```python
from build123d import *

# Parameters (mm, degrees)
F1_DEPTH = 63.5
F0_W     = 25.4
F0_H     = 19.05
F2_DEPTH = 25.4
F3_DEPTH = 7.9375
F5_R     = 6.35


with BuildPart() as f1:
    # F0 (on Front) → F1 (new body, symmetric)
    with BuildSketch(Plane.XZ):
        Polygon((41.275, -9.525), (41.275, 9.525), (22.225, 9.525), (-41.275, 9.525), (-41.275, -9.525), align=None)
    extrude(amount=F1_DEPTH, both=True)

    # F0 (on Front) → F2 (join, symmetric)
    with BuildSketch(Plane.XZ):
        with BuildLine():
            Line((57.15, 42.8752), (60.325, 42.8752))
            Line((60.325, 42.8752), (60.325, 61.9252))
            Line((60.325, 61.9252), (57.15, 61.9252))
            add(Edge.make_bspline(
                [(55.1509005081, 61.8679390466), (55.8211077358, 61.8945082476), (56.4875740772, 61.9136481218), (57.15, 61.9252)],
                knots=[109.7218611873, 109.7218611873, 109.7218611873, 109.7218611873, 111.5045361635, 111.5045361635, 111.5045361635, 111.5045361635], degree=3))
            ThreePointArc((55.1509005081, 61.8679390466), (31.7573418607, 50.9787015717), (22.225, 27.0002))
            Line((22.225, 27.0002), (22.225, 9.525))
            Line((22.225, 9.525), (41.275, 9.525))
            Line((41.275, 9.525), (41.275, 27.0002))
            ThreePointArc((41.275, 27.0002), (45.9246798487, 38.2255201513), (57.15, 42.8752))
        make_face()
        with Locations((73.025, 52.4002)):
            Rectangle(F0_W, F0_H)
    extrude(amount=F2_DEPTH, both=True)

    # F0 (on Front) → F3 (join, symmetric)
    with BuildSketch(Plane.XZ):
        with BuildLine():
            ThreePointArc((22.225, 27.0002), (31.7573418607, 50.9787015717), (55.1509005081, 61.8679390466))
            add(Edge.make_bspline(
                [(-41.275, 9.525), (-41.5217901281, 30.4529584249), (13.9003161981, 60.2326313083), (55.1509005081, 61.8679390466)],
                knots=[0, 0, 0, 0, 109.7218611873, 109.7218611873, 109.7218611873, 109.7218611873], degree=3))
            Line((-41.275, 9.525), (22.225, 9.525))
            Line((22.225, 9.525), (22.225, 27.0002))
        make_face()
    extrude(amount=F3_DEPTH, both=True)

    # F0 (on Front) → F4 (revolve)
    with BuildSketch(Plane.XZ):
        Polygon((85.725, 38.1), (111.125, 38.1), (111.125, 66.675), (85.725, 66.675), (85.725, 61.9252), (85.725, 42.8752), align=None)
    revolve(axis=Axis((85.725, 0, 52.3875), (0, 0, 1)))

    # F5
    f5_edges = [f1.edges().sort_by_distance(p)[0] for p in [
        (41.275, -63.5, 0),
        (-41.275, -63.5, 0),
        (41.275, 63.5, 0),
        (-41.275, 63.5, 0),
    ]]
    fillet(f5_edges, radius=F5_R)


solid = f1.part
```
The listing builds one solid part. Answer for the finished solid, in the listing's coordinates (mm). A direction names the side the tool comes from. Give positions to 0.01 mm unless a question says otherwise; leave off trailing zeros. Loops run counter-clockwise (first coordinate to the right, second up) from the corner with the lowest first, then second, coordinate; pieces in that order, holes last. Notation, with made-up numbers: M 38.25,37 L 80.25,37 A22 ccw 80.25,70 Z; hole C -8.5,-0.5 d5. An arc over 180 degrees is marked long. One line per item, written item: value.
1. Find the intervals of material crossed by probe 1 along Z at (x, y) = (17, -23) (3 decimals); probe 2 along X at (y, z) = (-47.5, 1.5) (3 decimals); probe 3 along Z at (x, y) = (76.5, -6) (3 decimals), in increasing order.
Found:
probe 1: -9.525 to 9.525
probe 2: -41.275 to 41.275
probe 3: 38.1 to 66.675
2. Each of these flat-tipped pins is pushed along its axis until it touches: P1, Ø19, axis at y = 19, z = 21, coming from the -X side (3 decimals); P2, Ø14.5, axis at x = 70, y = -11.5, coming from the -Z side; P3, Ø6, axis at x = -3.5, y = -11.5, coming from the +Z side (3 decimals); P4, Ø12, axis at x = 38, z = 13, coming from the -Y side. Where does it stop, or does it pass through?
Found:
P1: x = 22.225
P2: z = 38.1
P3: z = 9.525
P4: y = -63.5
3. Section B-B on y = 47.5 is taken. Determine the outline of the cut face in (x, z) (3 decimals).
Found:
outline: M -41.275,-9.525 L 41.275,-9.525 L 41.275,9.525 L -41.275,9.525 Z
4. For faces 4 (the face through (22.225, -17, 18)), 5 (the face through (86, 0, 38.1)), 6 (the face through (46, 25.4, 42)), 7 (the face through (45.8, -0.4, 38.1)), determine the directions among +Z, -Z, +X, -X, +Y, -Y from which every point of the face is accessible in a straight line to the end or side of a thin tool.
Found:
face 4: +Z, -X, -Y
face 5: -Z, +X, +Y, -Y
face 6: +Z, +X, -X, +Y
face 7: -Z, +Y, -Y
5. For a pull along X with two mould halves and no side action, classify faces 1 (the face through (60, 2, 42.875)), 2 (the face through (0, -63.5, 0)), 3 (the face through (39.464, -61.59, 0.133)) as pulls with the +X half, pulls with the -X half, needs draft (parallel to the pull), parting line crosses it, or undercut.
Found:
face 1: undercut
face 2: needs draft
face 3: pulls with the +X half
6. Section C-C on x = 98 is taken. Determine the outline of the cut face in (y, z) (3 decimals).
Found:
outline: M -22.237,38.1 L 22.237,38.1 L 22.237,66.675 L -22.237,66.675 Z
7. Section A-A on z = 5.5 is taken. Determine the outline of the cut face in (x, y) (3 decimals), plus the area to 3 significant figures.
Found:
outline: M -41.275,-57.15 A6.35 ccw -34.925,-63.5 L 34.925,-63.5 A6.35 ccw 41.275,-57.15 L 41.275,57.15 A6.35 ccw 34.925,63.5 L -34.925,63.5 A6.35 ccw -41.275,57.15 Z
area: 10,400 mm^2
